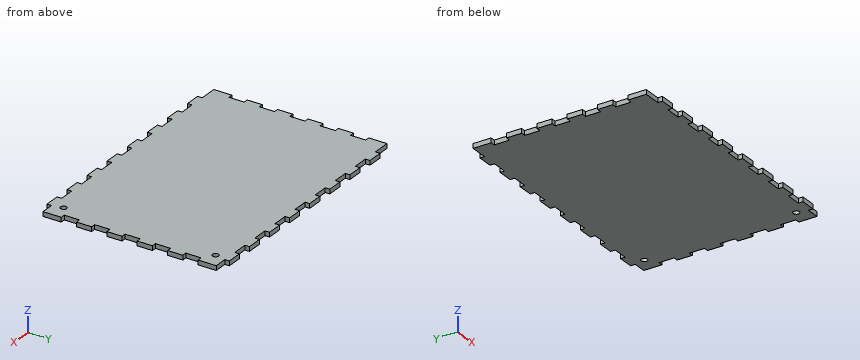
Autodesk Inventor part; units mm, degrees
ref_plane "YZ Plane" through (0, 0, 0) normal (1, 0, 0) x (0, 1, 0)
ref_plane "XZ Plane" through (0, 0, 0) normal (0, 1, 0) x (-1, 0, 0)
ref_plane "XY Plane" through (0, 0, 0) normal (0, 0, 1) x (1, 0, 0)
sketch "Esquisse1" plane through (0, 0, 0) normal (0, 0, 1) x (1, 0, 0)
  line L0 (87.3006, 60.3174) -> (87.3006, 48.3174)
  line L1 (87.3006, 38.3174) -> (87.3006, 28.3174)
  line L2 (84.3006, 48.3174) -> (84.3006, 38.3174)
  line L3 (84.3006, 48.3174) -> (87.3006, 48.3174)
  line L4 (84.3006, 38.3174) -> (87.3006, 38.3174)
  line L5 (84.3006, 28.3174) -> (84.3006, 18.3174)
  line L6 (84.3006, 28.3174) -> (87.3006, 28.3174)
  line L7 (78.8006, 60.3174) -> (87.3006, 60.3174)
  line L8 (68.8006, 63.3174) -> (78.8006, 63.3174)
  line L9 (78.8006, 63.3174) -> (78.8006, 60.3174)
  line L10 (58.8006, 60.3174) -> (68.8006, 60.3174)
  line L11 (68.8006, 63.3174) -> (68.8006, 60.3174)
  line L12 (48.8006, 63.3174) -> (58.8006, 63.3174)
  line L13 (58.8006, 63.3174) -> (58.8006, 60.3174)
  line L14 (48.8006, 63.3174) -> (48.8006, 60.3174)
  line L15 (38.8006, 63.3174) -> (38.8006, 60.3174)
  line L16 (18.8006, 60.3174) -> (28.8006, 60.3174)
  line L17 (28.8006, 63.3174) -> (38.8006, 63.3174)
  line L18 (28.8006, 63.3174) -> (28.8006, 60.3174)
  line L19 (38.8006, 60.3174) -> (48.8006, 60.3174)
  line L20 (87.3006, 18.3174) -> (87.3006, 8.3174)
  line L21 (87.3006, -21.6826) -> (87.3006, -31.6826)
  line L22 (87.3006, -1.6826) -> (87.3006, -11.6826)
  line L23 (87.3006, -41.6826) -> (87.3006, -53.6826)
  line L24 (84.3006, -31.6826) -> (84.3006, -41.6826)
  line L25 (84.3006, -31.6826) -> (87.3006, -31.6826)
  line L26 (48.8006, -56.6826) -> (58.8006, -56.6826)
  line L27 (58.8006, -56.6826) -> (58.8006, -53.6826)
  line L28 (58.8006, -53.6826) -> (68.8006, -53.6826)
  line L29 (68.8006, -56.6826) -> (68.8006, -53.6826)
  line L30 (68.8006, -56.6826) -> (78.8006, -56.6826)
  line L31 (78.8006, -56.6826) -> (78.8006, -53.6826)
  line L32 (78.8006, -53.6826) -> (87.3006, -53.6826)
  line L33 (84.3006, -41.6826) -> (87.3006, -41.6826)
  line L34 (84.3006, -21.6826) -> (87.3006, -21.6826)
  line L35 (84.3006, -11.6826) -> (84.3006, -21.6826)
  line L36 (84.3006, -11.6826) -> (87.3006, -11.6826)
  line L37 (84.3006, 8.3174) -> (84.3006, -1.6826)
  line L38 (84.3006, 8.3174) -> (87.3006, 8.3174)
  line L39 (84.3006, 18.3174) -> (87.3006, 18.3174)
  line L40 (84.3006, -1.6826) -> (87.3006, -1.6826)
  line L41 (-1.1994, 60.3174) -> (8.8006, 60.3174)
  line L42 (-21.1994, 60.3174) -> (-11.1994, 60.3174)
  line L43 (-11.1994, 63.3174) -> (-11.1994, 60.3174)
  line L44 (-11.1994, 63.3174) -> (-1.1994, 63.3174)
  line L45 (-1.1994, 63.3174) -> (-1.1994, 60.3174)
  line L46 (8.8006, 63.3174) -> (8.8006, 60.3174)
  line L47 (18.8006, 63.3174) -> (18.8006, 60.3174)
  line L48 (8.8006, 63.3174) -> (18.8006, 63.3174)
  line L49 (38.8006, -56.6826) -> (38.8006, -53.6826)
  line L50 (38.8006, -53.6826) -> (48.8006, -53.6826)
  line L51 (28.8006, -56.6826) -> (28.8006, -53.6826)
  line L52 (28.8006, -56.6826) -> (38.8006, -56.6826)
  line L53 (18.8006, -53.6826) -> (28.8006, -53.6826)
  line L54 (18.8006, -56.6826) -> (18.8006, -53.6826)
  line L55 (8.8006, -56.6826) -> (8.8006, -53.6826)
  line L56 (8.8006, -56.6826) -> (18.8006, -56.6826)
  line L57 (-1.1994, -53.6826) -> (8.8006, -53.6826)
  line L58 (-1.1994, -56.6826) -> (-1.1994, -53.6826)
  line L59 (-11.1994, -56.6826) -> (-11.1994, -53.6826)
  line L60 (-11.1994, -56.6826) -> (-1.1994, -56.6826)
  line L61 (-21.1994, -53.6826) -> (-11.1994, -53.6826)
  line L62 (-21.1994, -56.6826) -> (-21.1994, -53.6826)
  line L63 (-31.1994, -56.6826) -> (-31.1994, -53.6826)
  line L64 (-31.1994, -56.6826) -> (-21.1994, -56.6826)
  line L65 (-41.1994, -53.6826) -> (-31.1994, -53.6826)
  line L66 (48.8006, -56.6826) -> (48.8006, -53.6826)
  line L67 (-82.6994, 28.3174) -> (-82.6994, 38.3174)
  line L68 (-82.6994, 48.3174) -> (-82.6994, 60.3174)
  line L69 (-79.6994, 38.3174) -> (-79.6994, 48.3174)
  line L70 (-79.6994, 48.3174) -> (-82.6994, 48.3174)
  line L71 (-79.6994, 38.3174) -> (-82.6994, 38.3174)
  line L72 (-79.6994, 18.3174) -> (-79.6994, 28.3174)
  line L73 (-79.6994, 28.3174) -> (-82.6994, 28.3174)
  line L74 (-41.1994, 60.3174) -> (-31.1994, 60.3174)
  line L75 (-21.1994, 63.3174) -> (-21.1994, 60.3174)
  line L76 (-31.1994, 63.3174) -> (-31.1994, 60.3174)
  line L77 (-41.1994, 63.3174) -> (-41.1994, 60.3174)
  line L78 (-51.1994, 63.3174) -> (-41.1994, 63.3174)
  line L79 (-51.1994, 63.3174) -> (-51.1994, 60.3174)
  line L80 (-61.1994, 60.3174) -> (-51.1994, 60.3174)
  line L81 (-61.1994, 63.3174) -> (-61.1994, 60.3174)
  line L82 (-71.1994, 63.3174) -> (-61.1994, 63.3174)
  line L83 (-71.1994, 63.3174) -> (-71.1994, 60.3174)
  line L84 (-82.6994, 60.3174) -> (-71.1994, 60.3174)
  line L85 (-31.1994, 63.3174) -> (-21.1994, 63.3174)
  line L86 (-82.6994, 8.3174) -> (-82.6994, 18.3174)
  line L87 (-82.6994, -53.6826) -> (-82.6994, -41.6826)
  line L88 (-82.6994, -31.6826) -> (-82.6994, -21.6826)
  line L89 (-82.6994, -11.6826) -> (-82.6994, -1.6826)
  line L90 (-79.6994, 18.3174) -> (-82.6994, 18.3174)
  line L91 (-79.6994, -41.6826) -> (-79.6994, -31.6826)
  line L92 (-79.6994, -31.6826) -> (-82.6994, -31.6826)
  line L93 (-79.6994, -41.6826) -> (-82.6994, -41.6826)
  line L94 (-79.6994, -21.6826) -> (-79.6994, -11.6826)
  line L95 (-79.6994, -11.6826) -> (-82.6994, -11.6826)
  line L96 (-79.6994, -1.6826) -> (-79.6994, 8.3174)
  line L97 (-79.6994, -21.6826) -> (-82.6994, -21.6826)
  line L98 (-79.6994, 8.3174) -> (-82.6994, 8.3174)
  line L99 (-79.6994, -1.6826) -> (-82.6994, -1.6826)
  line L100 (-41.1994, -56.6826) -> (-41.1994, -53.6826)
  line L101 (-51.1994, -56.6826) -> (-41.1994, -56.6826)
  line L102 (-51.1994, -56.6826) -> (-51.1994, -53.6826)
  line L103 (-61.1994, -53.6826) -> (-51.1994, -53.6826)
  line L104 (-71.1994, -56.6826) -> (-61.1994, -56.6826)
  line L105 (-71.1994, -56.6826) -> (-71.1994, -53.6826)
  line L106 (-82.6994, -53.6826) -> (-71.1994, -53.6826)
  line L107 (-61.1994, -56.6826) -> (-61.1994, -53.6826)
  point P0 (0, 0)
extrude "Extrusion1" add sketch "Esquisse1" along normal blind 3
hole "Perçage1" at (77.3006, 53.3174, 3) direction (0, 0, -1) diameter 4 end through all
hole "Perçage2" at (77.3006, -46.6826, 3) direction (0, 0, -1) diameter 4 end through all
properties part number "fond"
Verification items for the finished model (mm, model axes). Coordinates: 2 decimals unless noted, no trailing zeros. Order: outer loops, then holes, each group sorted by start corner. A loop starts at its lowest first (then second) coordinate and runs counter-clockwise, first axis right, second up. Notation, with made-up numbers: (61, 56) -> (114, 56) arc R5 ccw to (114, 64) -> close; hole circle Ø3 at (-13, 86.25). An arc over 180 degrees is marked (long way). Answer as CSV lines item,"result". Start each with the question number.
1) Cross-section at B-B, the plane x = 24.5. Record the boundary of the cut face in (y, z), then the cut area to 3 significant figures.
2) Cross-section at C-C, the plane z = 0.8. Give the number of separate pieces and of enclosed holes in the cut face, then the cut area to 3 significant figures.
3) Gauge pin test, flat ends, axial feed: pin 1 Ø1.5 at (x, z) = (-35.5, 1.5) entering from +Y; pin 2 Ø0.9 at (y, z) = (62, 1.5) entering from -X; pin 3 Ø0.9 at (x, z) = (-37.5, 1.5) entering from -Y. Record the tip position at first contact, or that the pin passes through.
4) Cross-section at A-A, the plane y = -36. Record the boundary of the cut face in (x, z).
5) Material ranges on L1, parallel to Y at x = 79, z = 1.4; L2, parallel to X at y = -35.5, z = 1.2; L3, parallel to Y at x = -33, z = 0.3, recorded low to high. Write a range as [from, to].
Conclusion:
1,outline,"(-53.68, 0) -> (60.32, 0) -> (60.32, 3) -> (-53.68, 3) -> close"
1,area,"342 mm²"
2,separate pieces,"1"
2,enclosed holes,"2"
2,area,"19,500 mm²"
3,pin 1,"stops at y = 60.32"
3,pin 2,"stops at x = -71.2"
3,pin 3,"stops at y = -53.68"
4,outline,"(-79.7, 0) -> (84.3, 0) -> (84.3, 3) -> (-79.7, 3) -> close"
5,L1,"y = [-53.68, -47.74], [-45.63, 52.26], [54.37, 60.32]"
5,L2,"x = [-79.7, 84.3]"
5,L3,"y = [-53.68, 60.32]"
